Could you check a few things on this model? Use its own coordinates, in mm. Give positions to 0.01 mm unless a question says otherwise; leave off trailing zeros. Loops run counter-clockwise (first coordinate to the right, second up) from the corner with the lowest first, then second, coordinate; pieces in that order, holes last. Notation, with made-up numbers: (-15.75, 57.25) -> (30.25, 57.25) arc R29 ccw to (30.25, 79.25) -> close; hole circle Ø10 at (-28, 5.25). An arc over 180 degrees is marked (long way). Put each result on its own line as item: value.
```python
from build123d import *

# Parameters (mm, degrees)
F0_R     = 5.8001703578
F1_DEPTH = 5


with BuildPart() as f1:
    # F0 (on Top) → F1 (new body)
    with BuildSketch(Plane.XY):
        with BuildLine():
            ThreePointArc((-51.5878325652, 43.0670979278), (-43.6064509364, 39.8107528074), (-35.8466573247, 43.5646626824))
            ThreePointArc((-35.8466573247, 43.5646626824), (-33.9913764501, 46.7608427975), (-33.3468052575, 50.3998210098))
            ThreePointArc((-33.3468052575, 50.3998210098), (-34.5801317872, 55.3608197394), (-37.9929595743, 59.1667636721))
            ThreePointArc((-37.9929595743, 59.1667636721), (-52.0356668806, 57.2349793372), (-51.5878325652, 43.0670979278))
        make_face()
        with BuildLine():
            ThreePointArc((-40.1209657017, 47.1739723683), (-48.6369571368, 52.1172344713), (-38.9411621027, 50.3998210098))
            ThreePointArc((-38.9411621027, 50.3998210098), (-39.2453670685, 48.6824075484), (-40.1209657017, 47.1739723683))
        make_face(mode=Mode.SUBTRACT)
        with BuildLine():
            ThreePointArc((-33.3468052575, 50.3998210098), (-33.9913764501, 46.7608427975), (-35.8466573247, 43.5646626824))
            Line((-35.8466573247, 43.5646626824), (-11.0028552614, 22.586069771))
            ThreePointArc((-11.0028552614, 22.586069771), (-0.4004973799, 28.421312646), (11.3836651948, 25.6656703485))
            Line((11.3836651948, 25.6656703485), (-37.9929595743, 59.1667636721))
            ThreePointArc((-37.9929595743, 59.1667636721), (-34.5801317872, 55.3608197394), (-33.3468052575, 50.3998210098))
        make_face()
        with BuildLine():
            Line((-11.0028552614, 22.586069771), (-35.8466573247, 43.5646626824))
            ThreePointArc((-35.8466573247, 43.5646626824), (-43.6064509364, 39.8107528074), (-51.5878325652, 43.0670979278))
            Line((-51.5878325652, 43.0670979278), (-10.2889293891, 0))
            ThreePointArc((-10.2889293891, 0), (-14.9796236946, 11.1560494348), (-11.0028552614, 22.586069771))
        make_face()
        with BuildLine():
            ThreePointArc((11.3836651948, 25.6656703485), (-0.4004973799, 28.421312646), (-11.0028552614, 22.586069771))
            ThreePointArc((-11.0028552614, 22.586069771), (-14.9796236946, 11.1560494348), (-10.2889293891, 0))
            ThreePointArc((-10.2889293891, 0), (-9.3307459574, -0.923461232), (-8.3028313172, -1.7686166191))
            ThreePointArc((-8.3028313172, -1.7686166191), (9.4147958872, -3.4362525243), (18.7904441289, 11.6896373111))
            ThreePointArc((18.7904441289, 11.6896373111), (17.7735553067, 17.4615447103), (14.8453410404, 22.5384078277))
            ThreePointArc((14.8453410404, 22.5384078277), (13.2229979304, 24.2221357766), (11.3836651948, 25.6656703485))
        make_face()
        with BuildLine():
            ThreePointArc((7.4177247191, 11.6896373111), (0.0063621285, 6.5087384654), (-2.3136509097, 15.2487354792))
            ThreePointArc((-2.3136509097, 15.2487354792), (3.7960272887, 16.8705361568), (7.4177247191, 11.6896373111))
        make_face(mode=Mode.SUBTRACT)
        with BuildLine():
            ThreePointArc((18.7904441289, 11.6896373111), (9.4147958872, -3.4362525243), (-8.3028313172, -1.7686166191))
            Line((-8.3028313172, -1.7686166191), (39.4306997632, -37.9601014858))
            ThreePointArc((39.4306997632, -37.9601014858), (38.2144708977, -22.8923814768), (53.3235958963, -23.3716942143))
            Line((53.3235958963, -23.3716942143), (14.8453410404, 22.5384078277))
            ThreePointArc((14.8453410404, 22.5384078277), (17.7735553067, 17.4615447103), (18.7904441289, 11.6896373111))
        make_face()
        with BuildLine():
            ThreePointArc((53.3235958963, -23.3716942143), (38.2144708977, -22.8923814768), (39.4306997632, -37.9601014858))
            ThreePointArc((39.4306997632, -37.9601014858), (50.0643321154, -38.9609706715), (55.6913382216, -29.8828277773))
            ThreePointArc((55.6913382216, -29.8828277773), (55.0810295299, -26.4186877688), (53.3235958963, -23.3716942143))
        make_face()
        with Locations((45.5548754228, -29.8828277773)):
            Circle(F0_R, mode=Mode.SUBTRACT)
    extrude(amount=F1_DEPTH)


solid = f1.part
```
1. If we section it at A-A (x = -46.5): List the corners of the cut face in (y, z) for me.
Recorded:
outline: (37.76, 0) -> (46.1, 0) -> (46.1, 5) -> (37.76, 5) -> close; (54.7, 0) -> (60.68, 0) -> (60.68, 5) -> (54.7, 5) -> close
2. If we section it at B-B (z = 3.6): List the corners of the cut face in (x, y) for me, then the cut area to 3 significant figures.
Recorded:
outline: (-51.59, 43.07) -> (-10.29, 0) arc R16.89 ccw to (-8.3, -1.77) -> (39.43, -37.96) arc R10.14 ccw to (53.32, -23.37) -> (14.85, 22.54) arc R16.89 ccw to (11.38, 25.67) -> (-37.99, 59.17) arc R10.59 ccw to start; hole circle Ø10 at (-43.94, 50.4); hole circle Ø11.03 at (1.9, 11.69); hole circle Ø11.6 at (45.55, -29.88)
area: 3,360 mm^2
3. If we section it at C-C (x = 44): List the corners of the cut face in (y, z) for me, then the cut area to 3 significant figures.
Recorded:
outline: (-39.9, 0) -> (-35.47, 0) -> (-35.47, 5) -> (-39.9, 5) -> close; (-24.29, 0) -> (-12.25, 0) -> (-12.25, 5) -> (-24.29, 5) -> close
area: 82.4 mm^2
4. Thinking about a two-plate mould opening in Y: for faces 1 (the face through (13.25, 24.2, 2.46)), 2 (the face through (39.76, -29.63, 2.46)), 3 (the face through (-51.894, 57.4, 2.465)), which applies, pulls with the +Y half, pulls with the -Y half, needs draft (parallel to the pull), parting line crosses it, or undercut?
Recorded:
face 1: pulls with the +Y half
face 2: undercut
face 3: parting line crosses it
5. If we section it at D-D (y = 24): List the corners of the cut face in (x, z) for me, then the cut area to 3 significant figures.
Recorded:
outline: (-33.3, 0) -> (13.46, 0) -> (13.46, 5) -> (-33.3, 5) -> close
area: 234 mm^2
6. I need wall thicknesses on line 1 (X direction, y = -35, z = 1.15); line 2 (X direction, y = 50, z = 2.25); line 3 (Y direction, x = -1.5, z = 3.25). Which ranges of each line are inside material? Lowest first, please.
Recorded:
line 1: x = 35.53 to 42.82, 48.29 to 54.3
line 2: x = -54.53 to -48.93, -38.96 to -24.48
line 3: y = -6.93 to 7.35, 16.03 to 34.41
7. I'm going to push flat-ended pins straight in: pin 1 (10 mm diameter, centred on x = 1.9, y = 11.69, fed in from +Z); pin 2 (1 mm diameter, centred on x = 3.5, z = 0.5, fed in from -Y). Where does each tip first touch, or does it pass through?
Recorded:
pin 1: passes through
pin 2: stops at y = -11.1
